Autodesk Inventor part; units mm, degrees
ref_plane "YZ Plane" through (0, 0, 0) normal (1, 0, 0) x (0, 1, 0)
ref_plane "XZ Plane" through (0, 0, 0) normal (0, 1, 0) x (-1, 0, 0)
ref_plane "XY Plane" through (0, 0, 0) normal (0, 0, 1) x (1, 0, 0)
sketch "スケッチ1" plane through (0, 0, 0) normal (1, 0, 0) x (0, 1, 0)
  line L0 (-30, 15) -> (30, 15)
  line L1 (30, 15) -> (30, -15)
  line L2 (30, -15) -> (-30, -15)
  line L3 (-30, -15) -> (-30, 15)
  line L4 (-30, 15) -> (30, -15) construction
  line L5 (30, 15) -> (-30, -15) construction
  line L6 (27.7, 12.7) -> (-27.7, 12.7)
  line L7 (-27.7, 12.7) -> (-27.7, -12.7)
  line L8 (-27.7, -12.7) -> (27.7, -12.7)
  line L9 (27.7, -12.7) -> (27.7, 12.7)
  point P0 (0, 0)
  dimension "d0" = 60
  dimension "d1" = 30
  dimension "d2" = 2.3
extrude "押し出し1" add sketch "スケッチ1" along normal mid plane 163.5
sketch "スケッチ2" plane through (-81.75, 30, 15) normal (0, 1, 0) x (1, 0, 0)
  line L0 (163.5, 30) -> (0, 30)
  line L1 (163.5, 30) -> (163.5, 0)
  line L2 (0, 0) -> (0, 30)
  point P0 (16, 13)
  point P1 (147.5, 13)
  dimension "d14" = 17
  dimension "d15" = 17
  dimension "d16" = 16
  dimension "d17" = 16
hole "穴1" at (-65.75, 30, 2) at (65.75, 30, 2) direction (0, -1, 0) diameter 14 end through all
sketch "スケッチ5" plane through (-81.75, 27.7, -12.7) normal (0, 0, 1) x (1, 0, 0)
  circle A0 centre (34.1231, -45.7322) radius 5 construction
  point P0 (81.75, -27.7)
hole "穴2" at (-47.6269, -18.0322, -12.7) direction (0, 0, -1) diameter 8 end through all
properties part number "車軸受け3"
Could you check a few things on this model? Use its own coordinates, in mm. A direction names the side the tool comes from. Round coordinates to 2 decimals unless told otherwise and drop trailing zeros. Write each loop counter-clockwise with the first axis right and the second up, starting at its lowest first coordinate (ties: lowest second). Pieces come first, ordered by that corner, then holes. Notation, with made-up numbers: (67.25, 43) - (103.25, 43) arc R14 ccw to (103.25, 47) - close; hole circle Ø8 at (10, 0). An arc over 180 degrees is marked (long way). Use a Markdown table: item, result.
Q1. I want a section at B-B (x = -65.75). List the corners of the cut face in (y, z) for me.
Output values:
| item | result |
|---|---|
| outline | (-30, -15) - (30, -15) - (30, -5) - (27.7, -5) - (27.7, -12.7) - (-27.7, -12.7) - (-27.7, -5) - (-30, -5) - close; (-30, 9) - (-27.7, 9) - (-27.7, 12.7) - (27.7, 12.7) - (27.7, 9) - (30, 9) - (30, 15) - (-30, 15) - close |
Q2. I want a section at C-C (y = 1). List the corners of the cut face in (x, z) for me.
Output values:
| item | result |
|---|---|
| outline | (-81.75, -15) - (81.75, -15) - (81.75, -12.7) - (-81.75, -12.7) - close; (-81.75, 12.7) - (81.75, 12.7) - (81.75, 15) - (-81.75, 15) - close |
Q3. Thinking about a two-plate mould opening in X: for faces 1 (the flat face through (-81.75, -2, -13)), 2 (the flat face through (-1, 0, -12.7)), 3 (the cylindrical face through (-43.72, -17.17, -13.87)), which applies, released by +X, released by -X, zero draft, split by the parting line, or undercut?
Output values:
| item | result |
|---|---|
| face 1 | released by -X |
| face 2 | zero draft |
| face 3 | undercut |
Q4. I want a section at D-D (x = 42). List the corners of the cut face in (y, z) for me, plus the area to 3 significant figures.
Output values:
| item | result |
|---|---|
| outline | (-30, -15) - (30, -15) - (30, 15) - (-30, 15) - close; hole (-27.7, -12.7) - (27.7, -12.7) - (27.7, 12.7) - (-27.7, 12.7) - close |
| area | 393 mm2 |
Q5. For faces 4 (the flat face through (-1, -27.7, 0)), 5 (the cylindrical face through (-72.69, 28.83, 1.09)), which set-ups out of +Z, -Z, +X, -X, +Y, -Y let a thin tool reach every point of the face, with its end or its side?
Output values:
| item | result |
|---|---|
| face 4 | +X, -X |
| face 5 | +Y, -Y |
Q6. Please list where these lines run through material, in increasing order: L1, parallel to X at y = 29.05, z = 2; L2, parallel to Y at x = -23.5, z = -8.25; L3, parallel to Z at x = -65.75, y = 28.95.
Output values:
| item | result |
|---|---|
| L1 | -81.75 to -72.75, -58.75 to 58.75, 72.75 to 81.75 |
| L2 | -30 to -27.7, 27.7 to 30 |
| L3 | -15 to -5, 9 to 15 |
Q7. I want a section at A-A (z = 2). List the corners of the cut face in (x, y) for me, plus the area to 3 significant figures.
Output values:
| item | result |
|---|---|
| outline | (-81.75, -30) - (-72.75, -30) - (-72.75, -27.7) - (-81.75, -27.7) - close; (-81.75, 27.7) - (-72.75, 27.7) - (-72.75, 30) - (-81.75, 30) - close; (-58.75, -30) - (58.75, -30) - (58.75, -27.7) - (-58.75, -27.7) - close; (-58.75, 27.7) - (58.75, 27.7) - (58.75, 30) - (-58.75, 30) - close; (72.75, -30) - (81.75, -30) - (81.75, -27.7) - (72.75, -27.7) - close; (72.75, 27.7) - (81.75, 27.7) - (81.75, 30) - (72.75, 30) - close |
| area | 623 mm2 |
